Here's how the part is built. I have some questions about the finished solid (model axes, mm). A direction names the side the tool comes from. Round coordinates to 2 decimals unless told otherwise and drop trailing zeros. Answer as CSV lines item,"result".
```python
from build123d import *

# Parameters (mm, degrees)
EXTRUDE1_DEPTH = 609.6
EXTRUDE2_DEPTH = 612.086468922
SKETCH5_R      = 4.1656
EXTRUDE3_DEPTH = 445.930684208
SKETCH6_R      = 9.525
EXTRUDE4_DEPTH = 44.45


# Read off the part's stored shape, not the designer's step: 1515<1>
with BuildPart() as part:
    # Sketch1<2> → Extrude1 (new body)
    with BuildSketch(Plane(origin=(0, 0, 0), x_dir=(1, 0, 0), z_dir=(0, 1, 0))):
        Polygon((-6.7564, 4.364749804), (-6.7564, -4.364749804), (-14.986, -12.594349804), (-14.986, -4.064), (-19.05, -4.064), (-19.05, -19.05), (-4.064, -19.05), (-4.064, -14.986), (-13.067127258, -14.986), (-4.837527258, -6.7564), (4.837527258, -6.7564), (13.067127258, -14.986), (4.064, -14.986), (4.064, -19.05), (19.05, -19.05), (19.05, -4.064), (14.986, -4.064), (14.986, -12.594349804), (6.7564, -4.364749804), (6.7564, 4.364749804), (14.986, 12.594349804), (14.986, 4.064), (19.05, 4.064), (19.05, 19.05), (4.064, 19.05), (4.064, 14.986), (13.067127258, 14.986), (4.837527258, 6.7564), (-4.837527258, 6.7564), (-13.067127258, 14.986), (-4.064, 14.986), (-4.064, 19.05), (-19.05, 19.05), (-19.05, 4.064), (-14.986, 4.064), (-14.986, 12.594349804), align=None)
    extrude(amount=EXTRUDE1_DEPTH)

    # Sketch2 → Extrude2 (cut, through all)
    with BuildSketch(Plane.XY.offset(19.05)):
        Polygon((-19.05, 609.6), (19.05, 609.6), (19.05, 571.5), align=None)
        Polygon((19.05, 0), (19.05, 38.1), (-19.05, 0), align=None)
    extrude(amount=-EXTRUDE2_DEPTH, mode=Mode.SUBTRACT)

    # Sketch5 → Extrude3 (cut, through all)
    with BuildSketch(Plane(origin=(295.275, 295.275, 0), x_dir=(-0.7071067811865561, 0.7071067811865389, 5.599314837219468e-15), z_dir=(0.7071067811865389, 0.7071067811865561, 5.599314837219606e-15))):
        with Locations((415.947677993, 0)):
            Circle(SKETCH5_R)
    extrude3 = extrude(amount=-EXTRUDE3_DEPTH, mode=Mode.SUBTRACT)

    # Sketch6 → Extrude4 (cut)
    with BuildSketch(Plane(origin=(259.353975516, 259.353975516, 0), x_dir=(-0.7071067811865515, 0.7071067811865437, 0), z_dir=(0.7071067811865437, 0.7071067811865515, 0))):
        with Locations((415.947677993, 0)):
            Circle(SKETCH6_R)
    extrude4 = extrude(amount=EXTRUDE4_DEPTH, mode=Mode.SUBTRACT)

    # Mirror14: Extrude3, Extrude4 across plane
    add(extrude3.mirror(Plane.ZX.offset(304.8)), mode=Mode.SUBTRACT)
    add(extrude4.mirror(Plane.ZX.offset(304.8)), mode=Mode.SUBTRACT)


solid = part.part
```
1. We'd pull the mould along X, two halves only. Please class faces 4 (the flat face through (-12, 301, 19.05)), 5 (the flat face through (0.18, 28.21, 0.12)), 6 (the flat face through (0.27, 590.28, 4.5)): pulls with the +X half, pulls with the -X half, needs draft (parallel to the pull), parting line crosses it, or undercut.
Evaluation:
face 4,"needs draft"
face 5,"undercut"
face 6,"pulls with the +X half"
2. For P1, Ø4.5, axis at y = 594.5, z = -1, coming from the -X side; P2, Ø3, axis at x = 8.5, z = 15, coming from the -Y side; P3, Ø5, axis at x = 1, z = 10, coming from the +Y side; P4, Ø4, axis at y = 216, z = 2, coming from the +X side, each with a flat end and sliding along its axis, tell me the tip position at first contact or that it passes through.
Evaluation:
P1,"stops at x = -6.76"
P2,"stops at y = 26.05"
P3,"passes through"
P4,"stops at x = 6.76"
3. If I drill on line 1 (X direction, y = 329, z = -6); line 2 (Z direction, x = -4.5, y = 56); line 3 (Z direction, x = -6.5, y = 51), over which ranges is the centre line in solid material (lowest first)? Write a range as [from, to].
Evaluation:
line 1,"x = [-19.05, -14.99], [-8.39, 8.39], [14.99, 19.05]"
line 2,"z = [-19.05, -14.99], [-6.76, 6.76], [14.99, 19.05]"
line 3,"z = [-19.05, -14.99], [-8.42, 8.42], [14.99, 19.05]"
4. Which directions (+Z, -Z, +X, -X, +Y, -Y) give clear straight access to the entire face, cutting with the end or side of a thin tool? Please do faces 1 (the flat face through (0.18, 581.39, 0.12)), 2 (the flat face through (0, 301, 6.756)), 3 (the flat face through (19.05, 301, 12)).
Evaluation:
face 1,"none"
face 2,"+Y, -Y"
face 3,"+Z, -Z, +X, +Y, -Y"
